```python
from build123d import *

# Parameters (mm, degrees)
SKETCH1_R              = 10
BOSS_EXTRUDE1_DEPTH    = 45
M10X1_0_TAPPED_HOLE1_D = 9


with BuildPart() as part:
    # Sketch1 → Boss-Extrude1 (new body, symmetric)
    with BuildSketch(Plane.XY):
        with BuildLine():
            Line((-18.047378541, 21.380711875), (-11.952621459, 8.619288125))
            ThreePointArc((-11.952621459, 8.619288125), (-10, 0), (-11.952621459, -8.619288125))
            Line((-11.952621459, -8.619288125), (-18.047378541, -21.380711875))
            ThreePointArc((-18.047378541, -21.380711875), (0, -50), (18.047378541, -21.380711875))
            Line((18.047378541, -21.380711875), (11.952621459, -8.619288125))
            ThreePointArc((11.952621459, -8.619288125), (10, 0), (11.952621459, 8.619288125))
            Line((11.952621459, 8.619288125), (18.047378541, 21.380711875))
            ThreePointArc((18.047378541, 21.380711875), (0, 50), (-18.047378541, 21.380711875))
        make_face()
        with Locations((0, 30)):
            Circle(SKETCH1_R, mode=Mode.SUBTRACT)
        with Locations((0, -30)):
            Circle(SKETCH1_R, mode=Mode.SUBTRACT)
    extrude(amount=BOSS_EXTRUDE1_DEPTH, both=True)

    # M10x1.0 Tapped Hole1 (through all)
    with Locations(Plane.XY.offset(45)):
        with Locations((0, 0)):
            Hole(M10X1_0_TAPPED_HOLE1_D / 2)


solid = part.part
```
Part model, mm, in its own coordinate system. A direction names the side the tool comes from. Round coordinates to 2 decimals unless told otherwise and drop trailing zeros. Write each loop counter-clockwise with the first axis right and the second up, starting at its lowest first coordinate (ties: lowest second). Pieces come first, ordered by that corner, then holes. Notation, with made-up numbers: M 84.25,14.5 L 90.25,14.5 A24 cw 90.25,45.5 Z; hole C -8,20 d8. An arc over 180 degrees is marked long. One line per question, with ' | ' between items.
(1) Pin check, flat tips, straight feed: pin 1 (12 mm diameter, centred on x = 6.5, z = -25.5, fed in from +Y); pin 2 (4 mm diameter, centred on y = -1, z = 31.5, fed in from -X); pin 3 (6 mm diameter, centred on y = 25, z = -30.5, fed in from -X). Stop position of each tip, or through.
Answer key:
pin 1: stops at y = 49.99 | pin 2: stops at x = -10.23 | pin 3: stops at x = -19.9
(2) Saw through at B-B on z = -17. Write the cut outline in (x, y).
Answer key:
outline: M -18.05,-21.38 A20 ccw long 18.05,-21.38 L 11.95,-8.62 A20 cw 11.95,8.62 L 18.05,21.38 A20 ccw long -18.05,21.38 L -11.95,8.62 A20 cw -11.95,-8.62 Z; hole C 0,-30 d20; hole C 0,30 d20; hole C 0,0 d9
(3) Saw through at A-A on x = 0. Write the cut outline in (y, z), then the cut area to 3 significant figures.
Answer key:
outline: M -50,-45 L -40,-45 L -40,45 L -50,45 Z; M -20,-45 L -4.5,-45 L -4.5,45 L -20,45 Z; M 4.5,-45 L 20,-45 L 20,45 L 4.5,45 Z; M 40,-45 L 50,-45 L 50,45 L 40,45 Z | area: 4,590 mm^2
(4) Saw through at D-D on x = 15.5. Write the cut outline in (y, z).
Answer key:
outline: M -42.64,-45 L -16.05,-45 L -16.05,45 L -42.64,45 Z; M 16.05,-45 L 42.64,-45 L 42.64,45 L 16.05,45 Z
(5) Probe line 1 along Y through (x, z) = (0, 4); line 2 along Y through (x, z) = (8.5, -18); line 3 along X through (y, z) = (-0.5, -25). List the from-to ranges inside material, lowest first.
Answer key:
line 1: y = -50 to -40, -20 to -4.5, 4.5 to 20, 40 to 50 | line 2: y = -48.1 to -35.27, -24.73 to 24.73, 35.27 to 48.1 | line 3: x = -10.01 to -4.47, 4.47 to 10.01
(6) 3-axis set-ups, long thin cutter, end or side, ignore diameter. For faces 1 (the face through (15, -15, 1)), 2 (the face through (-15, -15, 1)), 3 (the face through (-5, 1, -45)): which of +Z, -Z, +X, -X, +Y, -Y reach the whole face in a straight line?
Answer key:
face 1: +Z, -Z, +X | face 2: +Z, -Z, -X | face 3: -Z, +X, -X, +Y, -Y
(7) Two-plate mould, pull along X, no slides. Class faces 4 (the face through (-5, 1, 45)), 5 (the face through (-15, 15, 1)), 6 (the face through (0.59, 4.46, -0.63)): released by +X, released by -X, zero draft, split by the parting line, or undercut.
Answer key:
face 4: zero draft | face 5: released by -X | face 6: undercut
(8) Saw through at C-C on y = 30. Write the cut outline in (x, z), then the cut area to 3 significant figures.
Answer key:
outline: M -20,-45 L -10,-45 L -10,45 L -20,45 Z; M 10,-45 L 20,-45 L 20,45 L 10,45 Z | area: 1,800 mm^2
